Verification items for the finished model (mm, model axes). A direction names the side the tool comes from. Round coordinates to 2 decimals unless told otherwise and drop trailing zeros. Write each loop counter-clockwise with the first axis right and the second up, starting at its lowest first coordinate (ties: lowest second). Pieces come first, ordered by that corner, then holes. Notation, with made-up numbers: (85.5, -14.5) - (121.5, -14.5) arc R21 cw to (121.5, 23.5) - close; hole circle Ø3 at (42.5, 45). An arc over 180 degrees is marked (long way). Answer as a JSON object with one key per item and string values.
```python
from build123d import *

# Parameters (mm, degrees)
CROQUIS1_R              = 11.115
CROQUIS1_R_2            = 2.5
SALIENTE_EXTRUIR1_DEPTH = 6.35
CROQUIS3_R              = 2.5
CORTAR_EXTRUIR1_DEPTH   = 10
REDONDEO1_R             = 5


with BuildPart() as part:
    # Croquis1 → Saliente-Extruir1 (new body)
    with BuildSketch(Plane(origin=(0, 0, 0), x_dir=(0, 0, -1), z_dir=(1, 0, 0))):
        with BuildLine():
            Line((-30.06, -68.26), (-30.06, 1.76))
            ThreePointArc((-30.06, 1.76), (-32.696038969, 8.123961031), (-39.06, 10.76))
            Line((-39.06, 10.76), (-269.71, 10.76))
            Line((-269.71, 10.76), (-269.71, -30.77))
            Line((-269.71, -30.77), (-319.71, -30.77))
            Line((-319.71, -30.77), (-319.71, 10.76))
            Line((-319.71, 10.76), (-319.71, 68.26))
            Line((-319.71, 68.26), (21.06, 68.26))
            Line((21.06, 68.26), (76.54, 68.26))
            Line((76.54, 68.26), (76.54, -30.77))
            Line((76.54, -30.77), (30.06, -30.77))
            Line((30.06, -30.77), (30.06, -68.26))
            Line((30.06, -68.26), (-30.06, -68.26))
        make_face()
        with Locations((0, 43.26)):
            Circle(CROQUIS1_R, mode=Mode.SUBTRACT)
        with Locations((0, -36.51)):
            Circle(CROQUIS1_R, mode=Mode.SUBTRACT)
        with Locations((-243.18, 43.26)):
            Circle(CROQUIS1_R, mode=Mode.SUBTRACT)
        Circle(CROQUIS1_R_2, mode=Mode.SUBTRACT)
        with Locations((-67.59, 43.26)):
            Circle(CROQUIS1_R_2, mode=Mode.SUBTRACT)
        with Locations((-167.59, 43.26)):
            Circle(CROQUIS1_R_2, mode=Mode.SUBTRACT)
        with Locations((-132.59, 43.26)):
            Circle(CROQUIS1_R_2, mode=Mode.SUBTRACT)
        with Locations((-102.59, 43.26)):
            Circle(CROQUIS1_R_2, mode=Mode.SUBTRACT)
    extrude(amount=SALIENTE_EXTRUIR1_DEPTH)

    # Croquis3 → Cortar-Extruir1 (cut)
    with BuildSketch(Plane(origin=(6.35, 0, 0), x_dir=(0, 0, -1), z_dir=(1, 0, 0))):
        with Locations((-288.21, -22.77)):
            Circle(CROQUIS3_R)
        with Locations((-306.21, -22.77)):
            Circle(CROQUIS3_R)
        with Locations((-306.21, 22.78)):
            Circle(CROQUIS3_R)
        with Locations((-288.21, 22.78)):
            Circle(CROQUIS3_R)
        with Locations((45.04, -22.77)):
            Circle(CROQUIS3_R)
        with Locations((63.04, -22.77)):
            Circle(CROQUIS3_R)
        with Locations((45.04, 22.78)):
            Circle(CROQUIS3_R)
        with Locations((63.04, 22.78)):
            Circle(CROQUIS3_R)
        with Locations((-309.103398282, 57.653398282)):
            Circle(CROQUIS3_R)
        with Locations((65.933398282, 57.653398282)):
            Circle(CROQUIS3_R)
    extrude(amount=-CORTAR_EXTRUIR1_DEPTH, mode=Mode.SUBTRACT)

    # Redondeo1
    redondeo1_edges = [part.edges().sort_by_distance(p)[0] for p in [
        (3.175, -68.26, -30.06),
        (3.175, -68.26, 30.06),
        (3.175, 10.76, 269.71),
        (3.175, -30.77, 269.71),
        (3.175, -30.77, 319.71),
        (3.175, 68.26, 319.71),
        (3.175, 68.26, -76.54),
        (3.175, -30.77, -76.54),
    ]]
    fillet(redondeo1_edges, radius=REDONDEO1_R)


solid = part.part
```
Q1. Set-up check for faces 5 (the flat face through (3, -30.77, -51)), 6 (the cylindrical face through (3.131, 8.054, 32.626)), 7 (the flat face through (3, -30.77, 294)): record each of +Z, -Z, +X, -X, +Y, -Y from which the full face is reachable in a straight line by a thin tool's end or side.
Geometry check:
{"face 5": "-Z, +X, -X, -Y", "face 6": "+X, -X, -Y", "face 7": "+Z, +X, -X, -Y"}
Q2. Section check A-A, the plane y = -6.5. Record the cut outline in (x, z).
Geometry check:
{"outline": "(0, -76.54) - (6.35, -76.54) - (6.35, 30.06) - (0, 30.06) - close; (0, 269.71) - (6.35, 269.71) - (6.35, 319.71) - (0, 319.71) - close"}
Q3. Release check for a two-part mould opening along Y. For faces 1 (the flat face through (3, -47, -30.06)), 2 (the cylindrical face through (3.131, 39.003, 232.913)), 3 (the cylindrical face through (3.13, -27.14, -5.98)), 4 (the flat face through (3, 68.26, 124)) record: released by +Y, released by -Y, zero draft, split by the parting line, or undercut.
Geometry check:
{"face 1": "zero draft", "face 2": "undercut", "face 3": "undercut", "face 4": "released by +Y"}
Q4. Section check B-B, the plane z = 57. Record the cut outline in (x, y), then the cut area to 3 significant figures.
Geometry check:
{"outline": "(0, 10.76) - (6.35, 10.76) - (6.35, 68.26) - (0, 68.26) - close", "area": "365 mm2"}
Q5. Gauge pin test, flat ends, axial feed: P1, Ø1.9, axis at x = 4.5, z = 300, coming from the -Y side; P2, Ø6, axis at y = 0, z = 0, coming from the +X side. Record the tip position at first contact, or that the pin passes through.
Geometry check:
{"P1": "stops at y = -30.77", "P2": "stops at x = 6.35"}
Q6. Material ranges on line 1 along Y through (x, z) = (2, 0) (3 decimals); line 2 along Y through (x, z) = (3.5, 288.21); line 3 along Y through (x, z) = (3, 67.59), recorded low to high. Write a range as [from, to].
Geometry check:
{"line 1": "y = [-68.26, -47.625], [-25.395, -2.5], [2.5, 32.145], [54.375, 68.26]", "line 2": "y = [-30.77, -25.27], [-20.27, 20.28], [25.28, 68.26]", "line 3": "y = [10.76, 40.76], [45.76, 68.26]"}
Q7. Section check C-C, the plane x = 1.25. State how many separate pieces and enclosed holes the cut face has, then the cut area to 3 significant figures.
Geometry check:
{"separate pieces": "1", "enclosed holes": "18", "area": "30,100 mm2"}
